Model file for the job. Use its own axes, mm. A direction names the side the tool comes from. Coordinates: 2 decimals unless noted, no trailing zeros. Loops run counter-clockwise (first coordinate to the right, second up) from the corner with the lowest first, then second, coordinate; pieces in that order, holes last. Notation, with made-up numbers: (73.5, -11.75) -> (112.5, -11.75) arc R37 cw to (112.5, 27.25) -> close; hole circle Ø6 at (16, 14). An arc over 180 degrees is marked (long way). Use one line per item in the form item = value.
```python
from build123d import *

# Parameters (mm, degrees)
SKETCH1_R                    = 150
BOSS_EXTRUDE1_DEPTH          = 75
CHAMFER1_SIZE                = 10
BOSS_EXTRUDE2_START          = -75
BOSS_EXTRUDE2_DEPTH          = 10
CHAMFER2_SIZE                = 7
BOSS_EXTRUDE3_DEPTH          = 9
BOSS_EXTRUDE4_DEPTH          = 3.5
CIRPATTERN2_COUNT            = 4
CIRPATTERN2_COPY_1_DEPTH     = 9
CIRPATTERN2_COPY_2_DEPTH     = 9
CIRPATTERN2_COPY_3_DEPTH     = 9
CIRPATTERN2_COPY_4_DEPTH     = 3.5
CIRPATTERN2_COPY_5_DEPTH     = 3.5
CIRPATTERN2_COPY_6_DEPTH     = 3.5
CHAMFER2_OF_CIRPATTERN2_SIZE = 7
CUT_EXTRUDE2_START           = -60
CUT_EXTRUDE2_DEPTH           = 60
SKETCH7_R                    = 110
BOSS_EXTRUDE5_DEPTH          = 9
BOSS_EXTRUDE5_TAPER          = 45
SKETCH8_R                    = 15
BOSS_EXTRUDE6_DEPTH          = 20


with BuildPart() as part:
    # Sketch1 → Boss-Extrude1 (new body)
    with BuildSketch(Plane(origin=(0, 0, 0), x_dir=(1, 0, 0), z_dir=(0, 1, 0))):
        with Locations(Location((0, 0, 0), (0, 0, 270))):
            Circle(SKETCH1_R)
    extrude(amount=BOSS_EXTRUDE1_DEPTH)

    # Chamfer1
    chamfer1_edges = [part.edges().sort_by_distance(p)[0] for p in [
        (0, 75, -150),
    ]]
    chamfer(chamfer1_edges, length=CHAMFER1_SIZE)

    # Sketch2 → Boss-Extrude2 (add)
    with BuildSketch(Plane(origin=(0, 75, 0), x_dir=(1, 0, 0), z_dir=(0, 1, 0)).offset(BOSS_EXTRUDE2_START)):
        with BuildLine():
            Line((-145.236875483, 37.5), (-195.236875483, 37.5))
            Line((-195.236875483, 37.5), (-195.236875483, -37.5))
            Line((-195.236875483, -37.5), (-145.236875483, -37.5))
            ThreePointArc((-145.236875483, -37.5), (-150, 0), (-145.236875483, 37.5))
        make_face()
    boss_extrude2 = extrude(amount=BOSS_EXTRUDE2_DEPTH)

    # Chamfer2
    chamfer2_edges = [part.edges().sort_by_distance(p)[0] for p in [
        (-195.236875483, 5, -37.5),
        (-195.236875483, 5, 37.5),
    ]]
    chamfer(chamfer2_edges, length=CHAMFER2_SIZE)

    # Sketch4 → Boss-Extrude3 (add)
    with BuildSketch(Plane.XY.offset(37.5)):
        Polygon((-188.236875483, 10), (-145.236875483, 10), (-145.236875483, 65), (-170.556875483, 65), align=None)
    boss_extrude3 = extrude(amount=-BOSS_EXTRUDE3_DEPTH)

    # Sketch5 → Boss-Extrude4 (add)
    with BuildSketch(Plane(origin=(0, 10, 0), x_dir=(1, 0, 0), z_dir=(0, 1, 0))):
        Polygon((-183.173956068, -11.769233661), (-188.503341499, -9), (-193.566260913, -12.230766339), (-193.299794898, -18.230766339), (-187.970409467, -21), (-182.907490052, -17.769233661), align=None)
    boss_extrude4 = extrude(amount=BOSS_EXTRUDE4_DEPTH)

    # Mirror1: Boss-Extrude3, Boss-Extrude4 across plane
    add(boss_extrude3.mirror(Plane.XY))
    add(boss_extrude4.mirror(Plane.XY))

    # CirPattern2: Boss-Extrude2, Boss-Extrude3, Boss-Extrude4 ×4 about axis
    cirpattern2_axis = Axis((0, 0, 0), (0, 1, 0))
    add([boss_extrude2.rotate(cirpattern2_axis, i * 360 / CIRPATTERN2_COUNT) for i in range(1, CIRPATTERN2_COUNT)])
    add([boss_extrude3.rotate(cirpattern2_axis, i * 360 / CIRPATTERN2_COUNT) for i in range(1, CIRPATTERN2_COUNT)])
    add([boss_extrude4.rotate(cirpattern2_axis, i * 360 / CIRPATTERN2_COUNT) for i in range(1, CIRPATTERN2_COUNT)])

    # CirPattern2 copy 1 sketch → CirPattern2 copy 1 (add)
    with BuildSketch(Plane(origin=(-37.5, 0, 0), x_dir=(0, 0, -1), z_dir=(-1, 0, 0))):
        Polygon((-188.236875483, -10), (-145.236875483, -10), (-145.236875483, -65), (-170.556875483, -65), align=None)
    extrude(amount=-CIRPATTERN2_COPY_1_DEPTH)

    # CirPattern2 copy 2 sketch → CirPattern2 copy 2 (add)
    with BuildSketch(Plane(origin=(0, 0, 37.5), x_dir=(-1, 0, 0), z_dir=(0, 0, 1))):
        Polygon((-188.236875483, -10), (-145.236875483, -10), (-145.236875483, -65), (-170.556875483, -65), align=None)
    extrude(amount=-CIRPATTERN2_COPY_2_DEPTH)

    # CirPattern2 copy 3 sketch → CirPattern2 copy 3 (add)
    with BuildSketch(Plane(origin=(37.5, 0, 0), x_dir=(0, 0, 1), z_dir=(1, 0, 0))):
        Polygon((-188.236875483, -10), (-145.236875483, -10), (-145.236875483, -65), (-170.556875483, -65), align=None)
    extrude(amount=-CIRPATTERN2_COPY_3_DEPTH)

    # CirPattern2 copy 4 sketch → CirPattern2 copy 4 (add)
    with BuildSketch(Plane(origin=(0, 10, 0), x_dir=(0, 0, -1), z_dir=(0, 1, 0))):
        Polygon((-183.173956068, 11.769233661), (-188.503341499, 9), (-193.566260913, 12.230766339), (-193.299794898, 18.230766339), (-187.970409467, 21), (-182.907490052, 17.769233661), align=None)
    extrude(amount=CIRPATTERN2_COPY_4_DEPTH)

    # CirPattern2 copy 5 sketch → CirPattern2 copy 5 (add)
    with BuildSketch(Plane(origin=(0, 10, 0), x_dir=(-1, 0, 0), z_dir=(0, 1, 0))):
        Polygon((-183.173956068, 11.769233661), (-188.503341499, 9), (-193.566260913, 12.230766339), (-193.299794898, 18.230766339), (-187.970409467, 21), (-182.907490052, 17.769233661), align=None)
    extrude(amount=CIRPATTERN2_COPY_5_DEPTH)

    # CirPattern2 copy 6 sketch → CirPattern2 copy 6 (add)
    with BuildSketch(Plane.ZX.offset(10)):
        Polygon((-183.173956068, 11.769233661), (-188.503341499, 9), (-193.566260913, 12.230766339), (-193.299794898, 18.230766339), (-187.970409467, 21), (-182.907490052, 17.769233661), align=None)
    extrude(amount=CIRPATTERN2_COPY_6_DEPTH)

    # Chamfer2 of CirPattern2
    chamfer2_of_cirpattern2_edges = [part.edges().sort_by_distance(p)[0] for p in [
        (-37.5, 5, 195.236875483),
        (37.5, 5, 195.236875483),
        (195.236875483, 5, 37.5),
        (195.236875483, 5, -37.5),
        (37.5, 5, -195.236875483),
        (-37.5, 5, -195.236875483),
    ]]
    chamfer(chamfer2_of_cirpattern2_edges, length=CHAMFER2_OF_CIRPATTERN2_SIZE)

    # Sketch6 → Cut-Extrude2 (cut)
    with BuildSketch(Plane(origin=(0, 75, 0), x_dir=(1, 0, 0), z_dir=(0, 1, 0)).offset(CUT_EXTRUDE2_START)):
        with BuildLine():
            Line((-112.583302492, -65), (-129.903810568, -75))
            ThreePointArc((-129.903810568, -75), (-106.066017178, -106.066017178), (-75, -129.903810568))
            Line((-75, -129.903810568), (-65, -112.583302492))
            ThreePointArc((-65, -112.583302492), (-91.923881554, -91.923881554), (-112.583302492, -65))
        make_face()
    extrude(amount=CUT_EXTRUDE2_DEPTH, mode=Mode.SUBTRACT)

    # Sketch7 → Boss-Extrude5 (add)
    with BuildSketch(Plane(origin=(0, 75, 0), x_dir=(1, 0, 0), z_dir=(0, 1, 0))):
        Circle(SKETCH7_R)
    extrude(amount=BOSS_EXTRUDE5_DEPTH, taper=BOSS_EXTRUDE5_TAPER)

    # Sketch8 → Boss-Extrude6 (add)
    with BuildSketch(Plane(origin=(0, 84, 0), x_dir=(1, 0, 0), z_dir=(0, 1, 0))):
        with Locations(Location((0, 0, 0), (0, 0, 270))):
            Circle(SKETCH8_R)
    extrude(amount=BOSS_EXTRUDE6_DEPTH)


solid = part.part
```
Q1. Wall check: line 1 along Z through (x, y) = (155, 38); line 2 along Y through (x, z) = (47, -77). Give the ranges that are in metal, low to high.
Result:
line_1 = -37.5 to -28.5, 28.5 to 37.5
line_2 = 0 to 84
Q2. Band-saw the part on A-A, the plane x = 0. Write the cut outline in (y, z), and give its area (3 significant figures).
Result:
outline = (0, -195.24) -> (10, -195.24) -> (10, -150) -> (65, -150) -> (75, -140) -> (75, -110) -> (84, -101) -> (84, -15) -> (104, -15) -> (104, 15) -> (84, 15) -> (84, 101) -> (75, 110) -> (75, 140) -> (65, 150) -> (10, 150) -> (10, 195.24) -> (0, 195.24) -> close
area = 25,800 mm2
Q3. Pin check, flat tips, straight feed: pin 1 Ø12.5 at (x, y) = (-163, 41.5) entering from -Z; pin 2 Ø12 at (x, y) = (45, 60) entering from +Z; pin 3 Ø8 at (y, z) = (51, -48.5) entering from -X. Stop position of each tip, or through.
Result:
pin_1 = -37.5
pin_2 = 144.84
pin_3 = -143.25
Q4. Which spindle directions (+Z, -Z, +X, -X, +Y, -Y) get a long thin tool onto all of the face, cutting with end or side? Do faces 4 (the face through (15, 13.5, -188)), 5 (the face through (-33, 65, 158)), 6 (the face through (-163, 38, 28.5)), 7 (the face through (-121.12, 44.58, 69.93)). Say none if no direction does.
Result:
face_4 = -Z, +Y
face_5 = +Z, -X, +Y
face_6 = -X, +Y
face_7 = +Z, +Y
Q5. Mould opens along X. For faces 1 (the face through (105.272, 32.045, 106.854)), 2 (the face through (15, 13.5, 188)), 3 (the face through (-163, 38, -28.5)) say: released by +X, released by -X, zero draft, split by the parting line, or undercut.
Result:
face_1 = released by +X
face_2 = undercut
face_3 = zero draft
